from build123d import *

# Parameters (mm, degrees)
SKETCH1_W           = 110
SKETCH1_H           = 40
BOSS_EXTRUDE1_DEPTH = 26.1
SKETCH2_W           = 6.5
SKETCH2_H           = 6.8
CUT_EXTRUDE1_DEPTH  = 41
SKETCH3_W           = 65
SKETCH3_H           = 40
CUT_EXTRUDE2_DEPTH  = 20
SKETCH5_R           = 1.5
CUT_EXTRUDE3_DEPTH  = 27.1
FILLET1_R           = 5
SKETCH8_W           = 20
SKETCH8_H           = 40
CUT_EXTRUDE4_DEPTH  = 3
SKETCH9_W           = 40
SKETCH9_H           = 80
BOSS_EXTRUDE3_DEPTH = 7
SKETCH10_R          = 1.5
CUT_EXTRUDE5_DEPTH  = 7


with BuildPart() as part:
    # Sketch1 → Boss-Extrude1 (new body)
    with BuildSketch(Plane.XY):
        with Locations((5.766423358, -6.605839416)):
            Rectangle(SKETCH1_W, SKETCH1_H)
    extrude(amount=BOSS_EXTRUDE1_DEPTH)

    # Sketch2 → Cut-Extrude1 (cut, through all)
    with BuildSketch(Plane(origin=(0, 13.394160584, 0), x_dir=(1, 0, 0), z_dir=(0, 1, 0))):
        with Locations((57.516423358, -12.1)):
            Rectangle(SKETCH2_W, SKETCH2_H)
        Polygon((54.266423358, -19.8), (54.266423358, -15.5), (54.266423358, -8.7), (54.266423358, -4.4), (46.466423358, -4.4), (46.466423358, -19.8), align=None)
    extrude(amount=-CUT_EXTRUDE1_DEPTH, mode=Mode.SUBTRACT)

    # Sketch3 → Cut-Extrude2 (cut)
    with BuildSketch(Plane.XY.offset(26.1)):
        with Locations((3.266423358, -6.605839416)):
            Rectangle(SKETCH3_W, SKETCH3_H)
    extrude(amount=-CUT_EXTRUDE2_DEPTH, mode=Mode.SUBTRACT)

    # Sketch5 → Cut-Extrude3 (cut, through all)
    with BuildSketch(Plane.XY.offset(26.1)):
        with Locations((50.766423358, 6.394160584)):
            Circle(SKETCH5_R)
        with Locations((50.766423358, -8.605839416)):
            Circle(SKETCH5_R)
        with Locations((50.766423358, -23.605839416)):
            Circle(SKETCH5_R)
    extrude(amount=-CUT_EXTRUDE3_DEPTH, mode=Mode.SUBTRACT)

    # Fillet1
    fillet1_edges = [part.edges().sort_by_distance(p)[0] for p in [
        (35.766423358, -6.605839416, 26.1),
    ]]
    fillet(fillet1_edges, radius=FILLET1_R)

    # Sketch8 → Cut-Extrude4 (cut)
    with BuildSketch(Plane.XY.offset(26.1)):
        with Locations((-39.233576642, -6.605839416)):
            Rectangle(SKETCH8_W, SKETCH8_H)
    extrude(amount=-CUT_EXTRUDE4_DEPTH, mode=Mode.SUBTRACT)

    # Sketch9 → Boss-Extrude3 (add)
    with BuildSketch(Plane.XY.offset(23.1)):
        with Locations((-37.233576642, -6.605839416)):
            Rectangle(SKETCH9_W, SKETCH9_H)
    extrude(amount=-BOSS_EXTRUDE3_DEPTH)

    # Sketch10 → Cut-Extrude5 (cut)
    with BuildSketch(Plane.XY.offset(23.1)):
        with Locations((-24.233576642, 26.394160584)):
            Circle(SKETCH10_R)
        with Locations((-50.233576642, 26.394160584)):
            Circle(SKETCH10_R)
        with Locations((-52.233576642, -6.605839416)):
            Circle(SKETCH10_R)
        with Locations((-50.233576642, -39.605839416)):
            Circle(SKETCH10_R)
        with Locations((-24.233576642, -39.605839416)):
            Circle(SKETCH10_R)
    extrude(amount=-CUT_EXTRUDE5_DEPTH, mode=Mode.SUBTRACT)


solid = part.part
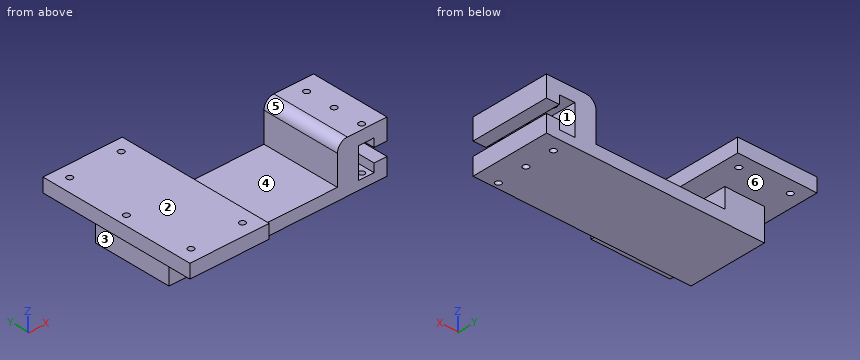
Model file for the job. Use its own axes, mm. Face numbers are marked on the shaded views. A direction names the side the tool comes from. Round coordinates to 2 decimals unless told otherwise and drop trailing zeros. Loops run counter-clockwise (first coordinate to the right, second up) from the corner with the lowest first, then second, coordinate; pieces in that order, holes last.
1. Band-saw the part on B-B, the plane x = -27. List the corners of the cut face in (y, z).
Check values:
outline: (-46.61, 16.1) - (33.39, 16.1) - (33.39, 23.1) - (-46.61, 23.1) - close; (-26.61, 0) - (13.39, 0) - (13.39, 6.1) - (-26.61, 6.1) - close
2. Mould opens along X. For the marked faces 1, 2 and 3 say: +X half, -X half, draft (parallel to the pull), parting line (faces both ways), or undercut.
Check values:
face 1: undercut
face 2: draft
face 3: -X half
3. Band-saw the part on D-D, the plane x = -42.5. List the corners of the cut face in (y, z).
Check values:
outline: (-46.61, 16.1) - (-26.61, 16.1) - (-26.61, 0) - (13.39, 0) - (13.39, 16.1) - (33.39, 16.1) - (33.39, 23.1) - (-46.61, 23.1) - close
4. Band-saw the part on C-C, the plane y = -0.5. List the corners of the cut face in (x, z).
Check values:
outline: (-57.23, 16.1) - (-49.23, 16.1) - (-49.23, 0) - (60.77, 0) - (60.77, 8.7) - (54.27, 8.7) - (54.27, 4.4) - (46.47, 4.4) - (46.47, 19.8) - (54.27, 19.8) - (54.27, 15.5) - (60.77, 15.5) - (60.77, 26.1) - (40.77, 26.1) arc R5 ccw to (35.77, 21.1) - (35.77, 6.1) - (-29.23, 6.1) - (-29.23, 16.1) - (-17.23, 16.1) - (-17.23, 23.1) - (-57.23, 23.1) - close
5. Band-saw the part on A-A, the plane z = 12. List the corners of the cut face in (x, y), and give its area (3 significant figures).
Check values:
outline: (-49.23, -26.61) - (-29.23, -26.61) - (-29.23, 13.39) - (-49.23, 13.39) - close; (35.77, -26.61) - (46.47, -26.61) - (46.47, 13.39) - (35.77, 13.39) - close
area: 1,230 mm2
6. Wall check: probe 1 along X at (y, z) = (11, 15.75); probe 2 along X at (y, z) = (10.5, 20.5); probe 3 along X at (y, z) = (-23, 13.5). Give the ranges that are in metal, low to high.
Check values:
probe 1: x = -49.23 to -29.23, 35.77 to 46.47, 54.27 to 60.77
probe 2: x = -57.23 to -17.23, 35.77 to 60.77
probe 3: x = -49.23 to -29.23, 35.77 to 46.47
7. Drop flat-ended pins along their axis: P1, Ø2.5, axis at x = 50.77, y = -23.61, coming from the +Z side; P2, Ø3.5, axis at x = -24.23, y = -39.61, coming from the +Z side; P3, Ø8, axis at y = -13.5, z = 6, coming from the -X side; P4, Ø3.5, axis at x = -50.23, y = -39.61, coming from the -Z side. Give the stop position or say it passes through.
Check values:
P1: passes through
P2: stops at z = 23.1
P3: stops at x = -49.23
P4: stops at z = 16.1
8. Tool access for the marked faces 4, 5 and 6: list every direction of +Z, -Z, +X, -X, +Y, -Y with a clear straight run to the whole face (end or side of a thin tool).
Check values:
face 4: +Y, -Y
face 5: +Z, +Y, -Y
face 6: none
